```python
from build123d import *

# Parameters (mm, degrees)
SKETCH1_W           = 70
SKETCH1_H           = 70
BOSS_EXTRUDE1_DEPTH = 2.5
SKETCH3_W           = 50
SKETCH3_H           = 50
BOSS_EXTRUDE4_DEPTH = 10
SKETCH5_W           = 40
SKETCH5_H           = 40
BOSS_EXTRUDE5_DEPTH = 5
SKETCH2_W           = 40
SKETCH2_H           = 40
CUT_EXTRUDE4_DEPTH  = 2.5
SKETCH6_W           = 30
SKETCH6_H           = 30
CUT_EXTRUDE5_DEPTH  = 15
SKETCH8_R           = 1.5
CUT_EXTRUDE6_DEPTH  = 5
SKETCH9_R           = 1.5
CUT_EXTRUDE7_DEPTH  = 5
FILLET1_R           = 2.5
FILLET2_R           = 2.5
FILLET3_R           = 2.5
SKETCH10_R          = 6.25
CUT_EXTRUDE12_DEPTH = 2.5


with BuildPart() as part:
    # Sketch1 → Boss-Extrude1 (new body)
    with BuildSketch(Plane.XY):
        with Locations((35, 35)):
            Rectangle(SKETCH1_W, SKETCH1_H)
    extrude(amount=BOSS_EXTRUDE1_DEPTH)

    # Sketch3 → Boss-Extrude4 (add)
    with BuildSketch(Plane(origin=(0, 0, 0), x_dir=(-1, 0, 0), z_dir=(0, 0, -1))):
        with Locations((-35, 35)):
            Rectangle(SKETCH3_W, SKETCH3_H)
    extrude(amount=BOSS_EXTRUDE4_DEPTH)

    # Sketch5 → Boss-Extrude5 (add)
    with BuildSketch(Plane(origin=(0, 0, -10), x_dir=(-1, 0, 0), z_dir=(0, 0, -1))):
        with Locations((-35, 35)):
            Rectangle(SKETCH5_W, SKETCH5_H)
    extrude(amount=BOSS_EXTRUDE5_DEPTH)

    # Sketch2 → Cut-Extrude4 (cut)
    with BuildSketch(Plane.XY.offset(2.5)):
        with Locations((35, 35)):
            Rectangle(SKETCH2_W, SKETCH2_H)
    extrude(amount=-CUT_EXTRUDE4_DEPTH, mode=Mode.SUBTRACT)

    # Sketch6 → Cut-Extrude5 (cut)
    with BuildSketch(Plane.XY):
        with Locations((35, 35)):
            Rectangle(SKETCH6_W, SKETCH6_H)
    extrude(amount=-CUT_EXTRUDE5_DEPTH, mode=Mode.SUBTRACT)

    # Sketch8 → Cut-Extrude6 (cut)
    with BuildSketch(Plane.XY):
        with Locations((52, 52)):
            Circle(SKETCH8_R)
        with Locations((52, 18)):
            Circle(SKETCH8_R)
        with Locations((18, 52)):
            Circle(SKETCH8_R)
        with Locations((18, 18)):
            Circle(SKETCH8_R)
    extrude(amount=-CUT_EXTRUDE6_DEPTH, mode=Mode.SUBTRACT)

    # Sketch9 → Cut-Extrude7 (cut)
    with BuildSketch(Plane(origin=(0, 0, -15), x_dir=(-1, 0, 0), z_dir=(0, 0, -1))):
        with Locations((-18, 18)):
            Circle(SKETCH9_R)
        with Locations((-52, 18)):
            Circle(SKETCH9_R)
        with Locations((-18, 52)):
            Circle(SKETCH9_R)
        with Locations((-52, 52)):
            Circle(SKETCH9_R)
    extrude(amount=-CUT_EXTRUDE7_DEPTH, mode=Mode.SUBTRACT)

    # Fillet1
    fillet1_edges = [part.edges().sort_by_distance(p)[0] for p in [
        (0, 70, 1.25),
        (70, 70, 1.25),
        (70, 0, 1.25),
        (0, 0, 1.25),
    ]]
    fillet(fillet1_edges, radius=FILLET1_R)

    # Fillet2
    fillet2_edges = [part.edges().sort_by_distance(p)[0] for p in [
        (15, 55, 1.25),
        (55, 55, 1.25),
    ]]
    fillet(fillet2_edges, radius=FILLET2_R)

    # Fillet3
    fillet3_edges = [part.edges().sort_by_distance(p)[0] for p in [
        (15, 15, 1.25),
        (55, 15, 1.25),
    ]]
    fillet(fillet3_edges, radius=FILLET3_R)

    # Sketch10 → Cut-Extrude12 (cut)
    with BuildSketch(Plane.XY.offset(2.5)):
        with Locations((52.5, 35)):
            Circle(SKETCH10_R)
    extrude(amount=-CUT_EXTRUDE12_DEPTH, mode=Mode.SUBTRACT)


solid = part.part
```
Check sheet for the modelled part. Datum: model origin and axes. Units: mm. A direction names the side the tool comes from. Give positions to 0.01 mm unless a question says otherwise; leave off trailing zeros. Write each loop counter-clockwise with the first axis right and the second up, starting at its lowest first coordinate (ties: lowest second). Pieces come first, ordered by that corner, then holes. Notation, with made-up numbers: (53.25, 17) -> (62.25, 17) arc R30 cw to (62.25, 43) -> close; hole circle Ø7 at (33.25, 15.5). An arc over 180 degrees is marked (long way). Use CSV: the item, a comma, the result in double quotes. Start each with the question number.
Q1. Tool access check on faces 4 (the flat face through (35, 20, -7)), 5 (the flat face through (18, 18, -5)), 6 (the flat face through (52, 18, -10)). Record the directions out of +Z, -Z, +X, -X, +Y, -Y that give a thin tool (end or side, any length) a straight path to the whole face; none if there is none.
Q2. Cross-section at C-C on x = 4.5. Enter the section's corners in (y, z), and give its area (3 significant figures).
Q3. Cross-section at A-A on y = 45. Enter the section's corners in (x, z), and give its area (3 significant figures).
Q4. Release check for a two-part mould opening along Y. For faces 1 (the flat face through (35, 10, -5)), 2 (the cylindrical face through (19.2, 51.1, -12.5)), 3 (the flat face through (3, 35, 0)) record: +Y half, -Y half, draft (parallel to the pull), parting line (faces both ways), or undercut.
Q5. Depth check by flat-ended pin: P1, Ø2.5, axis at x = 52.5, y = 18, coming from the +Z side; P2, Ø1.5, axis at y = 42.5, z = -1, coming from the -X side; P3, Ø0.9, axis at x = 18, y = 18, coming from the +Z side. Enter the tip coordinate at first touch or a pass-through.
Q6. Scan lines: line 1 along Y through (x, z) = (52, -3.7); line 2 along Y through (x, z) = (25, -7.5). Record each from-to range of solid material in increasing order.
Working result:
1,face 4,"+Z, -Z"
1,face 5,"+Z"
1,face 6,"-Z"
2,outline,"(0, 0) -> (70, 0) -> (70, 2.5) -> (0, 2.5) -> close"
2,area,"175 mm^2"
3,outline,"(0, 0) -> (10, 0) -> (10, -10) -> (15, -10) -> (15, -15) -> (20, -15) -> (20, 0) -> (15, 0) -> (15, 2.5) -> (0, 2.5) -> close; (50, -15) -> (55, -15) -> (55, -10) -> (60, -10) -> (60, 0) -> (70, 0) -> (70, 2.5) -> (55, 2.5) -> (55, 0) -> (50, 0) -> close"
3,area,"325 mm^2"
4,face 1,"-Y half"
4,face 2,"undercut"
4,face 3,"draft"
5,P1,"stops at z = 0"
5,P2,"stops at x = 10"
5,P3,"stops at z = -5"
6,line 1,"y = 10 to 16.5, 19.5 to 50.5, 53.5 to 60"
6,line 2,"y = 10 to 20, 50 to 60"
